```python
from build123d import *

# Parameters (mm, degrees)
F0_R     = 12.7
F1_DEPTH = 152.4
F2_R     = 15.875
F2_R_2   = 12.7
F3_DEPTH = 177.8
F4_R     = 19.05
F4_R_2   = 15.875
F5_DEPTH = 203.2
F6_R     = 22.225
F6_R_2   = 19.05
F7_DEPTH = 304.8
F8_R     = 15.875
F9_DEPTH = 25.4


with BuildPart() as f1:
    # F0 (on Front) → F1 (new body)
    with BuildSketch(Plane.XZ):
        Circle(F0_R)
    extrude(amount=F1_DEPTH)

    # F2 (on face) → F3 (join)
    with BuildSketch(Plane.XZ.offset(152.4)):
        Circle(F2_R)
        Circle(F2_R_2, mode=Mode.SUBTRACT)
        Circle(F2_R_2)
    extrude(amount=F3_DEPTH)

    # F4 (on face) → F5 (join)
    with BuildSketch(Plane.XZ.offset(330.2)):
        Circle(F4_R)
        Circle(F4_R_2, mode=Mode.SUBTRACT)
        Circle(F4_R_2)
    extrude(amount=F5_DEPTH)

    # F6 (on face) → F7 (join)
    with BuildSketch(Plane.XZ.offset(533.4)):
        Circle(F6_R)
        Circle(F6_R_2, mode=Mode.SUBTRACT)
        Circle(F6_R_2)
    extrude(amount=F7_DEPTH)

    # F8 (on Right) → F9 (cut)
    with BuildSketch(Plane.YZ):
        with Locations((-796.925, 0)):
            Circle(F8_R)
    extrude(amount=-F9_DEPTH, mode=Mode.SUBTRACT)


solid = f1.part
```
Source: CAD feature listing. Evaluate the final solid. Frame: model axes, mm. A direction names the side the tool comes from. Give positions to 0.01 mm unless a question says otherwise; leave off trailing zeros. Loops run counter-clockwise (first coordinate to the right, second up) from the corner with the lowest first, then second, coordinate; pieces in that order, holes last. Notation, with made-up numbers: (88, -26) - (128, -26) arc R24 cw to (128, -3) - close; hole circle Ø2 at (36, 69). An arc over 180 degrees is marked (long way). Use CSV: the item, a comma, the result in double quotes. Start each with the question number.
1. Section A-A (z = 0). Output: boundary loops of the cut face in (x, y) (3 decimals).
2. Pin query (flat end, axial travel): pin 1 (6 mm diameter, centred on x = 3.5, y = -139.5, fed in from +Z); pin 2 (6 mm diameter, centred on x = 13.5, z = -13.5, fed in from +Y); pin 3 (8 mm diameter, centred on y = -571, z = 6, fed in from +X). Return the tip coordinate at first contact, or that it passes through.
3. Section C-C (y = -225). Output: boundary loops of the cut face in (x, z) (3 decimals).
4. Section B-B (y = -493). Output: boundary loops of the cut face in (x, z).
5. Ray query, L1, parallel to Y at x = -5, z = 13; L2, parallel to Y at x = 19, z = 4.5; L3, parallel to Z at x = 2, y = -125. Return the intervals inside material, ascending.
6. Reachability of faces 1 (the flat face through (0, 0, 0)), 2 (the flat face through (0, -797, 0)), 3 (the flat face through (-7, -152.4, 11)) from +Z, -Z, +X, -X, +Y, -Y: full face, straight path, thin tool, end or side. Return the list, or none.
Response:
1,outline,"(-22.225, -838.2) - (22.225, -838.2) - (22.225, -533.4) - (19.05, -533.4) - (19.05, -330.2) - (15.875, -330.2) - (15.875, -152.4) - (12.7, -152.4) - (12.7, 0) - (-12.7, 0) - (-12.7, -152.4) - (-15.875, -152.4) - (-15.875, -330.2) - (-19.05, -330.2) - (-19.05, -533.4) - (-22.225, -533.4) - (-22.225, -781.05) - (0, -781.05) - (0, -812.8) - (-22.225, -812.8) - close"
2,pin 1,"z = 12.69"
2,pin 2,"y = -330.2"
2,pin 3,"x = 22.13"
3,outline,"circle Ø31.75 at (0, 0)"
4,outline,"circle Ø38.1 at (0, 0)"
5,L1,"-838.2 to -806.04, -787.81 to -152.4"
5,L2,"-838.2 to -533.4"
5,L3,"-12.54 to 12.54"
6,face 1,"+Z, -Z, +X, -X, +Y"
6,face 2,"-X"
6,face 3,"+Y"
